Solid Edge part; units mm, degrees
sketch "Sketch1" plane through (-74.5, 0, 0) normal (1, 0, 0) x (0, 1, 0)
  line L0 (80.9905, 16.7958) -> (106.9905, 16.7958)
  line L1 (106.9905, 28.7958) -> (106.9905, 16.7958)
  line L2 (80.9905, 28.7958) -> (106.9905, 28.7958)
  line L3 (80.9905, 16.7958) -> (80.9905, 28.7958)
  circle A0 centre (84.2905, 22.7958) radius 1.5
  circle A1 centre (103.6905, 22.7958) radius 1.5
extrude "Protrusion1" add sketch "Sketch1" along normal blind 5
sketch "Sketch2" plane through (-72, 93.9905, 28.7958) normal (0, 0, 1) x (0, 1, 0)
  circle A0 centre (0.0095, 0.15) radius 0.8
extrude "ExtrudedCutout_1" cut sketch "Sketch2" against normal blind 7
sketch "Sketch3" plane through (-69.5, 93.9905, 22.7958) normal (1, 0, 0) x (0, 1, 0)
  line L0 (-9.7, -3) -> (-13, -3)
  line L1 (-13, 3) -> (-13, -3)
  line L2 (-13, 3) -> (-9.7, 3)
  arc A0 (-9.7, 3) -> (-9.7, -3) centre (-9.7, 0) cw
  line L3 (9.7, 3) -> (13, 3)
  line L4 (13, 3) -> (13, -3)
  line L5 (13, -3) -> (9.7, -3)
  arc A1 (9.7, -3) -> (9.7, 3) centre (9.7, 0) cw
extrude "ExtrudedCutout_3" cut sketch "Sketch3" against normal blind 2.5
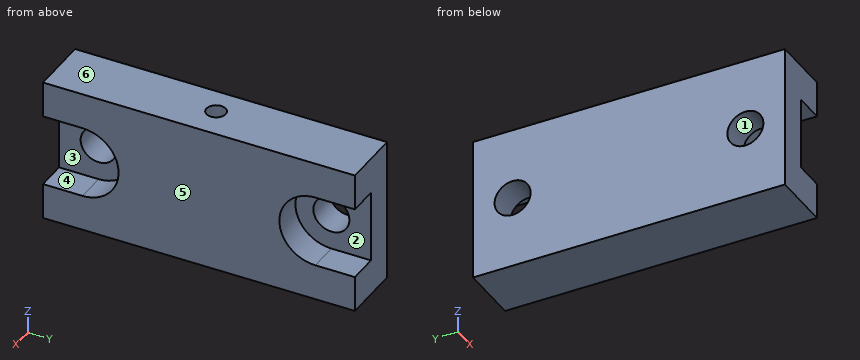
Here's how the part is built. I have some questions about the finished solid (model axes, mm). Face numbers are marked on the shaded views. A direction names the side the tool comes from. Coordinates: 2 decimals unless noted, no trailing zeros. Order: outer loops, then holes, each group sorted by start corner. A loop starts at its lowest first (then second) coordinate and runs counter-clockwise, first axis right, second up. Notation, with made-up numbers: M 9,-19.75 L 56,-19.75 A15 cw 56,-10.75 Z; hole C -9.75,83.25 d4. An arc over 180 degrees is marked long. Answer as CSV lines item,"result". Start each with the question number.
1. I want a section at B-B, the plane x = -69.9. Write out the boundary of the cut face in (y, z).
2. On a 3-axis mill with a long thin cutter (end or side, diameter ignored), from which of +Z, -Z, +X, -X, +Y, -Y can I reach the whole of each face in a straight line? I mean the marked faces 1 and 2. Say none if no direction works.
3. We'd pull the mould along Z, two halves only. Please class the marked faces 3, 4, 5 and 6: released by +Z, released by -Z, zero draft, split by the parting line, or undercut.
4. I want a section at A-A, the plane y = 94. Write out the boundary of the cut face in (x, z), and give its area (3 significant figures).
5. I need wall thicknesses on line 1 (Y direction, x = -72.25, z = 22.75); line 2 (X direction, y = 94, z = 24.5); line 3 (Z direction, x = -70.25, y = 104.5). Which ranges of each line are inside material? Lowest first, please. Write a range as [from, to].
6. I want a section at D-D, the plane y = 101.75. Write out the boundary of the cut face in (x, z).
7. I want a section at C-C, the plane z = 27.5. Write out the boundary of the cut face in (x, y), and give its area (3 significant figures).
8. For pin 1 (1.8 mm diameter, centred on y = 85, z = 23, fed in from +X), with a flat end and sliding along its axis, tell me the tip position at first contact or that it passes through.
Recorded:
1,outline,"M 80.99,16.8 L 106.99,16.8 L 106.99,19.8 L 103.69,19.8 A3 cw 103.69,25.8 L 106.99,25.8 L 106.99,28.8 L 80.99,28.8 L 80.99,25.8 L 84.29,25.8 A3 cw 84.29,19.8 L 80.99,19.8 Z"
2,face 1,"+X, -X"
2,face 2,"+X, +Y"
3,face 3,"undercut"
3,face 4,"undercut"
3,face 5,"zero draft"
3,face 6,"released by +Z"
4,outline,"M -74.5,16.8 L -69.5,16.8 L -69.5,28.8 L -71.35,28.8 L -71.35,21.8 L -72.95,21.8 L -72.95,28.8 L -74.5,28.8 Z"
4,area,"48.8 mm2"
5,line 1,"y = [80.99, 82.79], [85.79, 93.21], [94.79, 102.19], [105.19, 106.99]"
5,line 2,"x = [-74.5, -72.95], [-71.35, -69.5]"
5,line 3,"z = [16.8, 19.8], [25.8, 28.8]"
6,outline,"M -74.5,16.8 L -69.5,16.8 L -69.5,20.51 L -72,20.51 L -72,25.08 L -69.5,25.08 L -69.5,28.8 L -74.5,28.8 Z"
7,outline,"M -74.5,80.99 L -69.5,80.99 L -69.5,106.99 L -74.5,106.99 Z; hole C -72.15,94 d1.6"
7,area,"128 mm2"
8,pin 1,"stops at x = -72"
